Input: part model. Units: mm. Frame: model coordinates. Face numbers are marked on the shaded views. Round coordinates to 2 decimals unless told otherwise and drop trailing zeros. Loops run counter-clockwise (first coordinate to the right, second up) from the corner with the lowest first, then second, coordinate; pieces in that order, holes last.
1) Section D-D, the plane z = -1.75. Return loops of the section in (x, y).
2) Section A-A, the plane x = 5.5. Return loops of the section in (y, z), and give its area (4 significant figures).
3) Draft query along Z for the marked faces 1, 2 and 3. Return one class per face: pulls with the +Z half, pulls with the -Z half, needs draft (parallel to the pull), parting line crosses it, or undercut.
4) Section B-B, the plane z = 13.5. Return loops of the section in (x, y), and give its area (3 significant figures).
5) Ray query, line 1 along X through (y, z) = (-1.35, 13.5); line 2 along Z through (x, y) = (9, -0.05); line 3 along Y through (x, z) = (4.25, -0.75). Return the intervals inside material, ascending.
6) Section C-C, the plane y = 1.4. Return loops of the section in (x, z), and give its area (3 significant figures).
7) First-contact query: pin 1 (1.4 mm diameter, centred on y = -1.5, z = 8.5, fed in from -X); pin 2 (1.6 mm diameter, centred on x = 8, y = 1, fed in from -Z); pin 3 (0.6 mm diameter, centred on x = 12.5, y = -1, fed in from +Z). Flat tips, straight axial feed; report the tip coordinate or a pass-through.
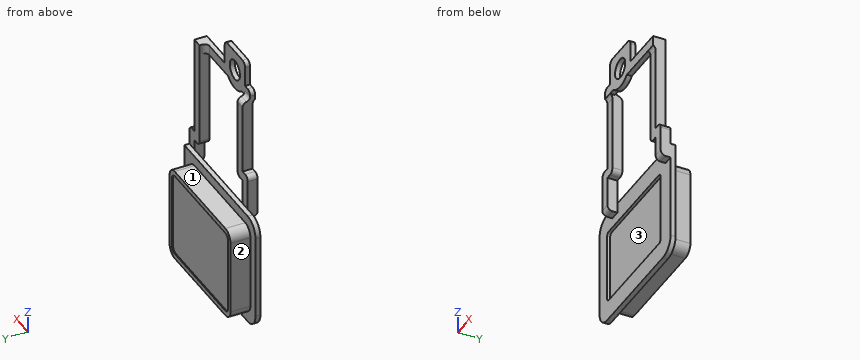
from build123d import *

# Parameters (mm, degrees)
SKETCH1_W                = 12
SKETCH1_H                = 9.5
BOSS_EXTRUDE1_DEPTH      = 2
SKETCH2_W                = 11
SKETCH2_H                = 8.5
CUT_EXTRUDE1_DEPTH       = 0.1
FILLET1_R                = 0.5
FILLET2_R                = 1
SKETCH3_W                = 14
SKETCH3_H                = 11.5
BOSS_EXTRUDE2_DEPTH      = 0.5
BOSS_EXTRUDE5_DEPTH      = 1
BOSS_EXTRUDE6_DEPTH      = 0.25
BOSS_EXTRUDE6_DEPTH_BACK = 0.25
SKETCH7_W                = 9.5
SKETCH7_H                = 1
BOSS_EXTRUDE7_DEPTH      = 0.5
CUT_EXTRUDE2_REACH       = 22.489
SKETCH10_R               = 1
FILLET4_R                = 0.5
FILLET5_R                = 0.5
FILLET6_R                = 1.5
SKETCH11_W               = 10.5
SKETCH11_H               = 7.5
CUT_EXTRUDE3_DEPTH       = 0.3
FILLET7_R                = 0.3


with BuildPart() as part:
    # Sketch1 → Boss-Extrude1 (new body)
    with BuildSketch(Plane(origin=(0, 0, 0), x_dir=(1, 0, 0), z_dir=(0, 1, 0))):
        with Locations((6, 4.75)):
            Rectangle(SKETCH1_W, SKETCH1_H)
    extrude(amount=BOSS_EXTRUDE1_DEPTH)

    # Sketch2 → Cut-Extrude1 (cut)
    with BuildSketch(Plane(origin=(0, 2, 0), x_dir=(1, 0, 0), z_dir=(0, 1, 0))):
        with Locations((6, 4.75)):
            Rectangle(SKETCH2_W, SKETCH2_H)
    extrude(amount=-CUT_EXTRUDE1_DEPTH, mode=Mode.SUBTRACT)

    # Fillet1
    fillet1_edges = [part.edges().sort_by_distance(p)[0] for p in [
        (0.5, 1.95, -0.5),
        (0.5, 1.95, -9),
        (11.5, 1.95, -9),
        (11.5, 1.95, -0.5),
    ]]
    fillet(fillet1_edges, radius=FILLET1_R)

    # Fillet2
    fillet2_edges = [part.edges().sort_by_distance(p)[0] for p in [
        (0, 1, -9.5),
        (12, 1, -9.5),
        (12, 1, 0),
        (0, 1, 0),
    ]]
    fillet(fillet2_edges, radius=FILLET2_R)

    # Sketch3 → Boss-Extrude2 (add)
    with BuildSketch(Plane.XZ):
        with Locations((6, -4.75)):
            Rectangle(SKETCH3_W, SKETCH3_H)
    extrude(amount=BOSS_EXTRUDE2_DEPTH)

    # Sketch6 → Boss-Extrude5 (add)
    with BuildSketch(Plane.XZ.offset(0.5)):
        Polygon((13, -0.5), (12, -0.5), (12, 2), (11, 2), (11, 13), (12, 13), (12, 3), (13, 3), align=None)
        Polygon((3.5, 12), (2.5, 12), (2.5, 4.5), (1.5, 4.5), (1.5, 0), (2.5, 0), (2.5, 3.5), (3.5, 3.5), align=None)
    extrude(amount=BOSS_EXTRUDE5_DEPTH)

    # Sketch7 → Boss-Extrude6 (add, two sides: drawn at the far end of the back side and taken through both)
    with BuildSketch(Plane.XZ.offset(1.5).offset(-BOSS_EXTRUDE6_DEPTH_BACK)):
        with Locations((7.25, 12.5)):
            Rectangle(SKETCH7_W, SKETCH7_H)
    extrude(amount=BOSS_EXTRUDE6_DEPTH + BOSS_EXTRUDE6_DEPTH_BACK)

    # Sketch9 → Boss-Extrude7 (add)
    with BuildSketch(Plane(origin=(0, -1.25, 0), x_dir=(1, 0, 0), z_dir=(0, 1, 0))):
        with BuildLine():
            Line((6.822875656, -12), (7.5, -12))
            Line((7.5, -12), (7.5, -15.5))
            Line((7.5, -15.5), (3.5, -15.5))
            Line((3.5, -15.5), (3.5, -12))
            Line((3.5, -12), (4.177124344, -12))
            ThreePointArc((4.177124344, -12), (5.5, -11.5), (6.822875656, -12))
        make_face()
    extrude(amount=-BOSS_EXTRUDE7_DEPTH)

    # Sketch10 → Cut-Extrude2 (cut, up to next)
    with BuildSketch(Plane(origin=(0, -1.25, 0), x_dir=(1, 0, 0), z_dir=(0, 1, 0)), mode=Mode.PRIVATE) as cut_extrude2_sk1:
        with Locations(Location((5.5, -13.5, 0), (0, 0, 270))):
            Circle(SKETCH10_R)
    cut_extrude2_tool1 = extrude(cut_extrude2_sk1.sketch, amount=-CUT_EXTRUDE2_REACH, mode=Mode.PRIVATE) & part.part
    add(cut_extrude2_tool1.solids().sort_by_distance((5.5, -1.25, 13.5))[0], mode=Mode.SUBTRACT)

    # Fillet4
    # the kernel refuses this fillet: 0.5 mm, written as the material it adds along each edge
    with BuildSketch(Plane(origin=(11, -1.25, 13), x_dir=(0, 1, 0), z_dir=(0, 0, -1))) as fillet4_piece_1:
        with BuildLine():
            CenterArc((FILLET4_R, -FILLET4_R), FILLET4_R, 90, 90)
            Line((0, -FILLET4_R), (0, 0))
            Line((0, 0), (FILLET4_R, 0))
        make_face()
    extrude(amount=1)
    with BuildSketch(Plane(origin=(3.5, -1.5, 12), x_dir=(0, 0, -1), z_dir=(-1, 0, 0))) as fillet4_piece_2:
        with BuildLine():
            CenterArc((0.433012702, 0.5), FILLET4_R, 210, 60)
            Line((0, 0.25), (0, 0))
            Line((0, 0), (0.433012702, 0))
        make_face()
    extrude(amount=1)
    # the kernel refuses this fillet: 0.5 mm, written as the material it takes off along each edge
    with BuildSketch(Plane(origin=(13, 0.75, 3), x_dir=(-1, 0, 0), z_dir=(0, -1, 0)), Plane(origin=(11, 0.75, 2), x_dir=(1, 0, 0), z_dir=(0, -1, 0)), Plane(origin=(14.25, -1.5, -0.5), x_dir=(0, 0, 1), z_dir=(-1, 0, 0)), Plane(origin=(3.5, 0.75, 3.5), x_dir=(0, 0, 1), z_dir=(0, -1, 0))) as fillet4_2_piece_1:
        with BuildLine():
            CenterArc((FILLET4_R, FILLET4_R), FILLET4_R, 180, 90)
            Line((0, FILLET4_R), (0, 0))
            Line((0, 0), (FILLET4_R, 0))
        make_face()
    extrude(amount=3.5, mode=Mode.SUBTRACT)
    with BuildSketch(Plane(origin=(4.75, -0.5, 12), x_dir=(0, -1, 0), z_dir=(-1, 0, 0)), Plane(origin=(1.5, 0.75, 4.5), x_dir=(1, 0, 0), z_dir=(0, -1, 0)), Plane(origin=(0.25, -1.5, 0), x_dir=(0, 0, 1), z_dir=(1, 0, 0))) as fillet4_2_piece_2:
        with BuildLine():
            CenterArc((FILLET4_R, -FILLET4_R), FILLET4_R, 90, 90)
            Line((0, -FILLET4_R), (0, 0))
            Line((0, 0), (FILLET4_R, 0))
        make_face()
    extrude(amount=3.5, mode=Mode.SUBTRACT)
    with BuildSketch(Plane(origin=(2.5, 0, 13), x_dir=(0, 0, -1), z_dir=(0, -1, 0)), Plane(origin=(3.5, 0, 15.5), x_dir=(0, 0, -1), z_dir=(0, -1, 0)), Plane(origin=(7.5, 0, 15.5), x_dir=(-1, 0, 0), z_dir=(0, -1, 0))) as fillet4_2_piece_3:
        with BuildLine():
            CenterArc((FILLET4_R, FILLET4_R), FILLET4_R, 180, 90)
            Line((0, FILLET4_R), (0, 0))
            Line((0, 0), (FILLET4_R, 0))
        make_face()
    extrude(amount=3, mode=Mode.SUBTRACT)

    # Fillet5
    # the kernel refuses this fillet: 0.5 mm, written as the material it adds along each edge
    with BuildSketch(Plane(origin=(3.5, -1.25, 12), x_dir=(0, 0.9991049126334705, -0.04230098759681056), z_dir=(-1, 0, 0))) as fillet5_piece_1:
        with BuildLine():
            CenterArc((0.479745195, -0.488977209), FILLET5_R, 102.053120737, 75.522487814)
            Line((-0.019807261, -0.467826716), (-0.069762507, -0.465711666))
            Line((-0.069762507, -0.465711666), (-0.049955246, 0.002115049))
            Line((-0.049955246, 0.002115049), (0.002115049, 0.049955246))
            ThreePointArc((0.002115049, 0.049955246), (0.251891278, 0.039379999), (0.364895035, 0.048897721))
            Line((0.364895035, 0.048897721), (0.375335958, 0))
        make_face()
    extrude(amount=1)
    with BuildSketch(Plane(origin=(12, -1.5, 12), x_dir=(0, -1, 0), z_dir=(-1, 0, 0))) as fillet5_piece_2:
        with BuildLine():
            CenterArc((0.5, -0.433012702), FILLET5_R, 120, 60)
            Line((0, -0.433012702), (0, 0))
            Line((0, 0), (0.25, 0))
        make_face()
    extrude(amount=1)

    # Fillet6
    fillet6_edges = [part.edges().sort_by_distance(p)[0] for p in [
        (-1, -0.25, 1),
        (-1, -0.25, -10.5),
        (13, -0.25, -10.5),
    ]]
    fillet(fillet6_edges, radius=FILLET6_R)

    # Sketch11 → Cut-Extrude3 (cut)
    with BuildSketch(Plane.XZ.offset(0.5)):
        with Locations((5.75, -4.75)):
            Rectangle(SKETCH11_W, SKETCH11_H)
    extrude(amount=-CUT_EXTRUDE3_DEPTH, mode=Mode.SUBTRACT)

    # Fillet7
    fillet7_edges = [part.edges().sort_by_distance(p)[0] for p in [
        (0.5, -0.35, -8.5),
        (0.5, -0.35, -1),
        (11, -0.35, -1),
        (11, -0.35, -8.5),
    ]]
    fillet(fillet7_edges, radius=FILLET7_R)


solid = part.part
Final values:
1. outline: (-1, -0.5) - (0.5, -0.5) - (0.5, -0.2) - (11, -0.2) - (11, -0.5) - (13, -0.5) - (13, 0) - (12, 0) - (12, 2) - (11.5, 2) - (11.5, 1.9) - (0.5, 1.9) - (0.5, 2) - (0, 2) - (0, 0) - (-1, 0) - close
2. outline: (-1.75, 11.5) - (-1.25, 11.5) - (-1.25, 12.5) - (-1.75, 12.5) - close; (-1.75, 14.5) - (-1.25, 14.5) - (-1.25, 15.5) - (-1.75, 15.5) - close; (-0.5, -10.5) - (0, -10.5) - (0, -9.5) - (2, -9.5) - (2, -9) - (1.9, -9) - (1.9, -0.5) - (2, -0.5) - (2, 0) - (0, 0) - (0, 1) - (-0.5, 1) - (-0.5, -1) - (-0.2, -1) - (-0.2, -8.5) - (-0.5, -8.5) - close
2. area: 22.65 mm2
3. face 1: pulls with the +Z half
3. face 2: needs draft
3. face 3: undercut
4. outline: (3.5, -1.75) - (4.5, -1.75) - (4.5, -1.25) - (3.5, -1.25) - close; (6.5, -1.75) - (7.5, -1.75) - (7.5, -1.25) - (6.5, -1.25) - close
4. area: 1.00 mm2
5. line 1: x = 3.5 to 4.5, 6.5 to 7.5
5. line 2: z = -10.5 to 1
5. line 3: y = -0.5 to 1.9
6. outline: (0, -8.5) arc R1 ccw to (1, -9.5) - (11, -9.5) arc R1 ccw to (12, -8.5) - (12, -1) arc R1 ccw to (11, 0) - (1, 0) arc R1 ccw to (0, -1) - close
6. area: 113 mm2
7. pin 1: stops at x = 2.5
7. pin 2: stops at z = -9.5
7. pin 3: stops at z = 3
